Input: part model. Units: mm. Frame: model coordinates. A direction names the side the tool comes from. Coordinates: 2 decimals unless noted, no trailing zeros. Loops run counter-clockwise (first coordinate to the right, second up) from the corner with the lowest first, then second, coordinate; pieces in that order, holes last. Notation, with made-up numbers: (72, 71.5) - (125, 71.5) arc R24 cw to (125, 93.5) - close; hole circle Ø9 at (87, 85). An arc over 180 degrees is marked (long way). Answer as CSV lines item,"result". Start each with the question number.
```python
from build123d import *

# Parameters (mm, degrees)
PAD_DEPTH       = 11
SKETCH001_R     = 9.75
POCKET_DEPTH    = 6
SKETCH002_R     = 5.5
POCKET001_DEPTH = 40
SKETCH003_R     = 9.75
POCKET002_DEPTH = 6
SKETCH004_R     = 2.25
POCKET003_DEPTH = 25
SKETCH005_R     = 1.5
POCKET004_DEPTH = 5


with BuildPart() as part:
    # Sketch → Pad (new body, symmetric)
    with BuildSketch(Plane.XZ):
        Polygon((-20.5, 40), (-20.5, 0), (13.5, 0), (13.5, 9), (20.8, 9), (20.8, 14), (13.5, 14), (13.5, 40), align=None)
    extrude(amount=PAD_DEPTH, both=True)

    # Sketch001 (on Face2 of Pad) → Pocket (cut)
    with BuildSketch(Plane(origin=(0, 0, 0), x_dir=(1, 0, 0), z_dir=(0, 0, -1))):
        Circle(SKETCH001_R)
    extrude(amount=-POCKET_DEPTH, mode=Mode.SUBTRACT)

    # Sketch002 (on Face12 of Pocket) → Pocket001 (cut)
    with BuildSketch(Plane(origin=(0, 0, 6), x_dir=(1, 0, 0), z_dir=(0, 0, -1))):
        Circle(SKETCH002_R)
    extrude(amount=-POCKET001_DEPTH, mode=Mode.SUBTRACT)

    # Sketch003 (on Face2 of Pocket001) → Pocket002 (cut)
    with BuildSketch(Plane(origin=(0, 0, 40), x_dir=(-1, 0, 0), z_dir=(0, 0, 1))):
        Circle(SKETCH003_R)
    extrude(amount=-POCKET002_DEPTH, mode=Mode.SUBTRACT)

    # Sketch004 (on Face5 of Pocket002) → Pocket003 (cut)
    with BuildSketch(Plane.XZ.offset(11)):
        with Locations((-15, 32.5)):
            Circle(SKETCH004_R)
        with Locations((-15, 7.5)):
            Circle(SKETCH004_R)
    extrude(amount=-POCKET003_DEPTH, mode=Mode.SUBTRACT)

    # Sketch005 (on Face11 of Pocket003) → Pocket004 (cut)
    with BuildSketch(Plane(origin=(0, 0, 9), x_dir=(1, 0, 0), z_dir=(0, 0, -1))):
        with Locations((16.95, 5)):
            Circle(SKETCH005_R)
        with Locations((16.95, -5)):
            Circle(SKETCH005_R)
    extrude(amount=-POCKET004_DEPTH, mode=Mode.SUBTRACT)


solid = part.part
```
Item 1: Draft query along X for faces 1 (the flat face through (17, 0, 9)), 2 (the cylindrical face through (-13.79, -0.154, 34.397)), 3 (the flat face through (-20.5, 0, 20)). Return one class per face: pulls with the +X half, pulls with the -X half, needs draft (parallel to the pull), parting line crosses it, or undercut.
Item 2: Section query C-C, the plane y = 6. Output: boundary loops of the cut face in (x, z).
Item 3: Section query D-D, the plane z = 18. Output: boundary loops of the cut face in (x, y), and give its area (3 significant figures).
Item 4: Contact query for flat-ended pins moving along their axis: P1, Ø1.8, axis at x = 16.95, y = 5, coming from the -Z side; P2, Ø7, axis at y = 3, z = 3.5, coming from the +X side; P3, Ø10, axis at x = 3, y = -1.5, coming from the +Z side; P4, Ø12.5, axis at x = 0, y = 0, coming from the -Z side. Output: stop coordinate, or through.
Item 5: Set-up query: faces 4 (the flat face through (-4, 4, 34)), 5 (the cylindrical face through (18.38, 4.55, 11.46)), 6 (the flat face through (17, 0, 14)), 7 (the flat face through (13.5, 0, 4)), 8 (the flat face through (4, 4, 6)). Return all of +Z, -Z, +X, -X, +Y, -Y with unobstructed straight access to the full face (end or side cutting, diameter ignored); none if empty.
Item 6: Section query A-A, the plane x = -15. Output: boundary loops of the cut face in (y, z), and give its area (3 significant figures).
Item 7: Material intervals for probe 1 along Y at (x, z) = (0, 35); probe 2 along X at (y, z) = (0, 26.5); probe 3 along X at (y, z) = (-1.5, 30.5), sorted ascending.
Item 8: Section query B-B, the plane z = 32.5. Output: boundary loops of the cut face in (x, y), and give its area (3 significant figures).
Response values:
1,face 1,"needs draft"
1,face 2,"undercut"
1,face 3,"pulls with the -X half"
2,outline,"(-20.5, 0) - (-7.69, 0) - (-7.69, 6) - (7.69, 6) - (7.69, 0) - (13.5, 0) - (13.5, 9) - (15.83, 9) - (15.83, 14) - (13.5, 14) - (13.5, 40) - (7.69, 40) - (7.69, 34) - (-7.69, 34) - (-7.69, 40) - (-20.5, 40) - close; (18.07, 9) - (20.8, 9) - (20.8, 14) - (18.07, 14) - close; hole circle Ø4.5 at (-15, 7.5); hole circle Ø4.5 at (-15, 32.5)"
3,outline,"(-20.5, -11) - (13.5, -11) - (13.5, 11) - (-20.5, 11) - close; hole circle Ø11 at (0, 0)"
3,area,"653 mm²"
4,P1,"passes through"
4,P2,"stops at x = 13.5"
4,P3,"stops at z = 34"
4,P4,"stops at z = 6"
5,face 4,"+Z"
5,face 5,"+Z, -Z"
5,face 6,"+Z, +X, +Y, -Y"
5,face 7,"-Z, +X, +Y, -Y"
5,face 8,"-Z"
6,outline,"(-11, 0) - (11, 0) - (11, 5.25) - (-11, 5.25) - close; (-11, 9.75) - (11, 9.75) - (11, 30.25) - (-11, 30.25) - close; (-11, 34.75) - (11, 34.75) - (11, 40) - (-11, 40) - close"
6,area,"682 mm²"
7,probe 1,"y = -11 to -9.75, 9.75 to 11"
7,probe 2,"x = -20.5 to -5.5, 5.5 to 13.5"
7,probe 3,"x = -20.5 to -16.03, -13.97 to -5.29, 5.29 to 13.5"
8,outline,"(-20.5, -11) - (-17.25, -11) - (-17.25, 11) - (-20.5, 11) - close; (-12.75, -11) - (13.5, -11) - (13.5, 11) - (-12.75, 11) - close; hole circle Ø11 at (0, 0)"
8,area,"554 mm²"
